```python
from build123d import *

# Parameters (mm, degrees)
SKETCH_1_R          = 20
EXTRUDE_1_DEPTH     = 20
SKETCH_2_R          = 2.5
CUT_EXTRUDE_1_DEPTH = 10
SKETCH_3_R          = 18
SKETCH_3_R_2        = 9
CUT_EXTRUDE_2_DEPTH = 2


with BuildPart() as part:
    # 草图1 → 凸台-拉伸1 (new body)
    with BuildSketch(Plane(origin=(0, 0, 0), x_dir=(1, 0, 0), z_dir=(0, 1, 0))):
        Circle(SKETCH_1_R)
    extrude(amount=EXTRUDE_1_DEPTH)

    # 草图2 → 切除-拉伸1 (cut)
    with BuildSketch(Plane(origin=(0, 20, 0), x_dir=(1, 0, 0), z_dir=(0, 1, 0))):
        Circle(SKETCH_2_R)
    extrude(amount=-CUT_EXTRUDE_1_DEPTH, mode=Mode.SUBTRACT)

    # 草图3 → 切除-拉伸2 (cut)
    with BuildSketch(Plane.XZ):
        Circle(SKETCH_3_R)
        Circle(SKETCH_3_R_2, mode=Mode.SUBTRACT)
    extrude(amount=-CUT_EXTRUDE_2_DEPTH, mode=Mode.SUBTRACT)


solid = part.part
```
Input: part model. Units: mm. Frame: model coordinates. A direction names the side the tool comes from. Round coordinates to 2 decimals unless told otherwise and drop trailing zeros. Order: outer loops, then holes, each group sorted by start corner. A loop starts at its lowest first (then second) coordinate and runs counter-clockwise, first axis right, second up. Notation, with made-up numbers: (58.5, 14.25) - (65.5, 14.25) arc R16 ccw to (65.5, 41.25) - close; hole circle Ø7 at (59, 13). An arc over 180 degrees is marked (long way). Answer in a Markdown table with one row per item.
Item 1: Pin query (flat end, axial travel): pin 1 (1.5 mm diameter, centred on y = 4, z = -6.5, fed in from +X); pin 2 (6 mm diameter, centred on x = -14, y = 16, fed in from +Z); pin 3 (1.5 mm diameter, centred on x = 1.5, z = -10, fed in from -Y). Return the tip coordinate at first contact, or that it passes through.
Model answer:
| item | result |
|---|---|
| pin 1 | stops at x = 19.16 |
| pin 2 | stops at z = 16.7 |
| pin 3 | stops at y = 2 |
Item 2: Reachability of faces 4 (the cylindrical face through (-0.54, 15.07, 2.44)), 5 (the flat face through (0, 0, 0)), 6 (the flat face through (-8.3, 2, 4.3)) from +Z, -Z, +X, -X, +Y, -Y: full face, straight path, thin tool, end or side. Return the list, or none.
Model answer:
| item | result |
|---|---|
| face 4 | +Y |
| face 5 | +Z, -Z, +X, -X, -Y |
| face 6 | -Y |
Item 3: Section query A-A (z = 0). Return the cut outline in (x, y), then the cut area to 3 significant figures.
Model answer:
| item | result |
|---|---|
| outline | (-20, 0) - (-18, 0) - (-18, 2) - (-9, 2) - (-9, 0) - (9, 0) - (9, 2) - (18, 2) - (18, 0) - (20, 0) - (20, 20) - (2.5, 20) - (2.5, 10) - (-2.5, 10) - (-2.5, 20) - (-20, 20) - close |
| area | 714 mm² |
Item 4: Line query: line 1 (Z direction, x = 0, y = 1.1); line 2 (Z direction, x = 0, y = 12.75). Output: solid intervals per line, ascending.
Model answer:
| item | result |
|---|---|
| line 1 | z = -20 to -18, -9 to 9, 18 to 20 |
| line 2 | z = -20 to -2.5, 2.5 to 20 |
Item 5: Section query D-D (x = 7). Return the cut outline in (y, z) (3 decimals).
Model answer:
| item | result |
|---|---|
| outline | (0, -18.735) - (20, -18.735) - (20, 18.735) - (0, 18.735) - (0, 16.583) - (2, 16.583) - (2, 5.657) - (0, 5.657) - (0, -5.657) - (2, -5.657) - (2, -16.583) - (0, -16.583) - close |
Item 6: Section query C-C (y = 5.25). Return the cut outline in (x, z).
Model answer:
| item | result |
|---|---|
| outline | circle Ø40 at (0, 0) |
Item 7: Mould query, pull axis Z, two halves, no side actions, for faces 1 (the flat face through (0, 10, 0)), 2 (the flat face through (-18, 0, -3)), 3 (the cylindrical face through (-4.336, 9.86, 19.524)). Classes: released by +Z, released by -Z, zero draft, split by the parting line, or undercut.
Model answer:
| item | result |
|---|---|
| face 1 | undercut |
| face 2 | zero draft |
| face 3 | split by the parting line |
Item 8: Section query B-B (x = 0). Return the cut outline in (y, z), then the cut area to 3 significant figures.
Model answer:
| item | result |
|---|---|
| outline | (0, -20) - (20, -20) - (20, -2.5) - (10, -2.5) - (10, 2.5) - (20, 2.5) - (20, 20) - (0, 20) - (0, 18) - (2, 18) - (2, 9) - (0, 9) - (0, -9) - (2, -9) - (2, -18) - (0, -18) - close |
| area | 714 mm² |
